Autodesk Inventor part; units mm, degrees
ref_plane "Work Plane1" through (6.5, 0, 0) normal (1, 0, 0) x (0, 1, 0)
ref_plane "XZ Plane" through (0, 0, 0) normal (0, 1, 0) x (-1, 0, 0)
ref_plane "XY Plane" through (0, 0, 0) normal (0, 0, 1) x (1, 0, 0)
sketch "Sketch1" plane through (0, 0, 0) normal (0, 1, 0) x (-1, 0, 0)
  circle A0 centre (0, 0) radius 6.5
  circle A1 centre (0, 0) radius 1.8
  dimension "d0" = 13
  dimension "d1" = 3.6
extrude "Extrusion1" add sketch "Sketch1" along normal blind 10
sketch "Sketch2" plane through (0, 10, 0) normal (0, 1, 0) x (1, 0, 0)
  point P0 (0, 0)
ref_plane "Work Plane1" through (6.5, 0, 0) normal (1, 0, 0) x (0, 1, 0)
sketch "Sketch3" plane through (6.5, 0, 0) normal (1, 0, 0) x (0, 1, 0)
  line L0 (10, -6.5) -> (10, 6.5)
  line L1 (10, -6.5) -> (22, -6.5)
  line L2 (22, -6.5) -> (22, 6.5)
  line L3 (22, 6.5) -> (10, 6.5)
  line L4 (10, 6.5) -> (10, -6.5)
  line L5 (0, -6.5) -> (0, 6.5)
  line L6 (10, -6.5) -> (0, -6.5)
  line L7 (0, -6.5) -> (0, 6.5)
  line L8 (0, 6.5) -> (10, 6.5)
  line L9 (10, 6.5) -> (10, -6.5)
  circle A0 centre (16, 0) radius 2
  point P0 (0, 0)
  point P1 (0, -6.5)
  point P2 (10, 6.5)
  point P3 (10, 6.5)
  dimension "d5" = 12
  dimension "d6" = 4
  dimension "d11" = 6
extrude "Extrusion2" add sketch "Sketch3" against normal up to surface contours L6 L5 L8 L0
extrude "Extrusion3" add sketch "Sketch3" along normal blind 7
sketch "Sketch5" plane through (0, 10, 0) normal (0, 1, 0) x (1, 0, 0)
  line L0 (3.4641, 0) -> (1.7321, -3)
  line L1 (1.7321, -3) -> (-1.7321, -3)
  line L2 (-1.7321, -3) -> (-3.4641, 0)
  line L3 (-3.4641, 0) -> (-1.7321, 3)
  line L4 (-1.7321, 3) -> (1.7321, 3)
  line L5 (1.7321, 3) -> (3.4641, 0)
  point P0 (0, 0)
  point P1 (0, 0)
  dimension "d12" = 6
extrude "Extrusion4" cut sketch "Sketch5" against normal blind 3
fillet "Fillet1" radius 4 2 edges at (10, 22, 6.5) (10, 22, -6.5)
sketch "Sketch6" plane through (6.5, 0, 0) normal (-1, 0, 0) x (0, 0, 1)
  circle A0 centre (0, 16) radius 2
  circle A1 centre (0, 16) radius 4
  point P0 (0, 0)
  dimension "d16" = 8
extrude "Extrusion5" cut sketch "Sketch6" against normal blind 2
chamfer "Chamfer1" distance 7 angle 45 1 edges at (13.5, 0, 0)
chamfer "Chamfer2" distance 3 angle 45 1 edges at (6.5, 10, 0)
properties part number "SpringConn"
Input: part model. Units: mm. Frame: model coordinates. A direction names the side the tool comes from. Round coordinates to 2 decimals unless told otherwise and drop trailing zeros. Loops run counter-clockwise (first coordinate to the right, second up) from the corner with the lowest first, then second, coordinate; pieces in that order, holes last. Notation, with made-up numbers: M 37.25,-34 L 54.25,-34 A23 cw 54.25,-21 Z; hole C 40,67 d11. An arc over 180 degrees is marked long. Answer in a Markdown table with one row per item. Add a question column.
1. Ray query, probe 1 along Z at (x, y) = (0, 4); probe 2 along Z at (x, y) = (9.5, 15); probe 3 along X at (y, z) = (13.5, 1.5). Return the intervals inside material, ascending.
2. Section B-B (y = 16). Output: boundary loops of the cut face in (x, z), and give its area (3 significant figures).
3. Contact query for flat-ended pins moving along their axis: pin 1 (1 mm diameter, centred on x = -1.5, z = 2, fed in from +Y); pin 2 (3 mm diameter, centred on x = -2, z = -2.5, fed in from +Y); pin 3 (3 mm diameter, centred on y = 4.5, z = -3, fed in from +X); pin 4 (10 mm diameter, centred on x = 7, y = 18.5, fed in from +Z). Output: stop coordinate, or through.
4. Set-up query: faces 1 (the face through (-4, 10, 0)), 2 (the face through (0, 9, -3)), 3 (the face through (7.311, 12.095, -0.867)), 4 (the face through (10.049, 20.859, 5.297)). Return all of +Z, -Z, +X, -X, +Y, -Y with unobstructed straight access to the full face (end or side cutting, diameter ignored); none if empty.
5. Section A-A (x = 7.5). Output: boundary loops of the cut face in (y, z).
6. Mould query, pull axis X, two halves, no side actions, for faces 5 (the face through (7, 9, -6.5)), 6 (the face through (8.5, 15, -2)), 7 (the face through (-2.6, 8.5, 1.5)), 8 (the face through (0, 9, 3)). Classes: released by +X, released by -X, zero draft, split by the parting line, or undercut.
7. Section C-C (z = 1.25). Output: boundary loops of the cut face in (x, y), and give its area (3 significant figures).
8. Section D-D (y = 5). Output: boundary loops of the cut face in (x, z).
Values follow:
| question | item | result |
|---|---|---|
| 1 | probe 1 | -6.5 to -1.8, 1.8 to 6.5 |
| 1 | probe 2 | -6.5 to -1.73, 1.73 to 6.5 |
| 1 | probe 3 | 8.5 to 13.5 |
| 2 | outline | M 6.5,-6.5 L 13.5,-6.5 L 13.5,-2 L 8.5,-2 L 8.5,-4 L 6.5,-4 Z; M 6.5,4 L 8.5,4 L 8.5,2 L 13.5,2 L 13.5,6.5 L 6.5,6.5 Z |
| 2 | area | 55.0 mm^2 |
| 3 | pin 1 | y = 7 |
| 3 | pin 2 | y = 10 |
| 3 | pin 3 | x = 12.5 |
| 3 | pin 4 | z = 6.5 |
| 4 | face 1 | +Z, -Z, -X, +Y |
| 4 | face 2 | +Y |
| 4 | face 3 | -X |
| 4 | face 4 | +Z, +X, -X, +Y |
| 5 | outline | M 1,-6.5 L 18,-6.5 A4 ccw 22,-2.5 L 22,2.5 A4 ccw 18,6.5 L 1,6.5 Z; hole C 16,0 d8 |
| 6 | face 5 | zero draft |
| 6 | face 6 | released by -X |
| 6 | face 7 | undercut |
| 6 | face 8 | undercut |
| 7 | outline | M -6.38,0 L -1.3,0 L -1.3,7 L -2.74,7 L -2.74,10 L -6.38,10 Z; M 1.3,0 L 6.5,0 L 13.5,7 L 13.5,14.44 L 8.5,14.44 L 8.5,12.2 L 5.7,12.2 L 3.5,10 L 2.74,10 L 2.74,7 L 1.3,7 Z; M 6.5,19.8 L 8.5,19.8 L 8.5,17.56 L 13.5,17.56 L 13.5,22 L 6.5,22 Z |
| 7 | area | 197 mm^2 |
| 8 | outline | M 0,-6.5 L 11.5,-6.5 L 11.5,6.5 L 0,6.5 A6.5 ccw Z; hole C 0,0 d3.6 |
